Autodesk Inventor part; units mm, degrees
ref_plane "Arbeitsebene1" through (-2.597, -2.44, -3) normal (0, 0, -1) x (0, 1, 0)
ref_plane "YZ Plane" through (0, 0, 0) normal (1, 0, 0) x (0, 1, 0)
ref_plane "XZ Plane" through (0, 0, 0) normal (0, 1, 0) x (-1, 0, 0)
sketch "Skizze1" plane through (0, 0, 0) normal (0, 0, 1) x (1, 0, 0)
  circle A0 centre (11.2246, 18.4558) radius 0.3325 construction
  circle A1 centre (11.2246, 18.4558) radius 1.1
  circle A2 centre (11.2246, 18.4558) radius 2.5
  point P0 (0, 0)
  dimension "d0" = 2.2
  dimension "d1" = 5
ref_plane "Arbeitsebene1" through (-2.597, -2.44, -3) normal (0, 0, -1) x (0, 1, 0)
extrude "Extrusion1" add sketch "Skizze1" against normal up to surface (3 mm away)
sketch "Skizze2" plane through (11.2246, 18.4558, 0) normal (0, 0, 1) x (1, 0, 0)
  line L0 (0, 0) -> (-2.8913, -4.716) construction
  line L1 (-2.8913, -4.716) -> (3.5184, 5.7389) construction
  line L2 (0, 0) -> (3.8461, -2.358) construction
  line L3 (-6.9448, -1.6658) -> (-1.6658, 6.9448)
  line L4 (-1.6658, 6.9448) -> (6.9448, 1.6658)
  line L5 (6.9448, 1.6658) -> (1.6658, -6.9448)
  line L6 (1.6658, -6.9448) -> (-6.9448, -1.6658)
  line L7 (-6.9448, -1.6658) -> (6.9448, 1.6658) construction
  line L8 (-1.6658, 6.9448) -> (1.6658, -6.9448) construction
  point P0 (-11.2246, -18.4558)
  dimension "d4" = 10.1
  dimension "d5" = 10.1
extrude "Extrusion2" add sketch "Skizze2" against normal blind 2
sketch "Skizze3" plane through (0, 0, 0) normal (0, 0, 1) x (1, 0, 0)
  line L0 (4.2798, 16.79) -> (9.5588, 25.4006)
  line L1 (12.8904, 11.511) -> (4.2798, 16.79)
  line L2 (18.1694, 20.1216) -> (12.8904, 11.511)
  line L3 (9.5588, 25.4006) -> (18.1694, 20.1216)
  line L4 (4.8948, 11.5894) -> (14.4118, 5.7548)
  line L5 (14.4118, 5.7548) -> (18.7104, 12.7664)
  line L6 (18.7104, 12.7664) -> (15.0398, 15.0168)
  line L7 (-1.5402, 15.5346) -> (18.7104, 12.7664) construction
  line L8 (14.4118, 5.7548) -> (2.7585, 22.5462) construction
  line L9 (4.8948, 11.5894) -> (7.0442, 15.0952)
  line L10 (12.8904, 11.511) -> (4.2798, 16.79)
  line L11 (7.0442, 15.0952) -> (12.8904, 11.511)
  line L12 (12.8904, 11.511) -> (15.0398, 15.0168)
  line L13 (18.1694, 20.1216) -> (12.8904, 11.511)
  point P0 (0, 0)
  point P1 (8.5851, 14.1505)
extrude "Extrusion3" add sketch "Skizze3" against normal blind 6 contours L1 L2 L6 L5 L4 L9
sketch "Skizze4" plane through (4.8948, 11.5894, -6) normal (-0.5227, -0.8525, 0) x (0.8525, -0.5227, 0)
  line L0 (-1.036, 2.1441) -> (1.7865, 3.0085)
  line L1 (0, 6) -> (11.1631, 6)
  line L2 (0, 6) -> (0, 0)
  line L3 (11.1631, 0) -> (0, 0)
  line L4 (11.1631, 6) -> (11.1631, 0)
  line L5 (0.7075, 3) -> (2.9075, 3)
  line L6 (1.3376, -2.7865) -> (1.3376, -9.7615)
  ellipse E0 centre (1.3376, -6.274) end of major axis (1.3376, 3) minor radius 7.5665
  point P0 (1.8845, 6)
extrude "Extrusion4" cut sketch "Skizze4" against normal up to surface (8.2244 mm away) contours L2 E0 L0 | L2 L3 E0 | L0 E0 L3 L2
sketch "Skizze5" plane through (0, 0, 0) normal (0, 0, 1) x (1, 0, 0)
  line L0 (4.2798, 16.79) -> (9.5588, 25.4006)
  line L1 (7.0442, 15.0952) -> (4.2798, 16.79)
  line L2 (7.0442, 15.0952) -> (4.8948, 11.5894)
  line L3 (4.8948, 11.5894) -> (14.4118, 5.7548)
  line L4 (14.4118, 5.7548) -> (18.7104, 12.7664)
  line L5 (18.7104, 12.7664) -> (15.0398, 15.0168)
  line L6 (18.1694, 20.1216) -> (15.0398, 15.0168)
  line L7 (9.5588, 25.4006) -> (18.1694, 20.1216)
  line L8 (7.0442, 15.0952) -> (4.8948, 11.5894)
  line L9 (7.0442, 15.0952) -> (8.6934, 9.2606)
  line L10 (10.7856, 7.9779) -> (4.8948, 11.5894)
  point P0 (0, 0)
extrude "Extrusion5" cut sketch "Skizze5" against normal blind 6 contours L9 L3 L2
chamfer "Fase1" distance 1 angle 45 1 edges at (12.9349, 11.4837, -6)
sketch "Skizze6" plane through (14.4118, 5.7548, -6) normal (-0.5227, -0.8525, 0) x (0.8525, -0.5227, 0)
  ellipse E0 centre (-9.8255, -6.274) end of major axis (-9.8255, -15.548) minor radius 7.5665 (-4.8984, 0.7642) -> (-6.7074, 2.1759) ccw
  ellipse E1 centre (-9.8255, -6.274) end of major axis (-9.8255, -15.548) minor radius 7.5665 (-6.7074, 2.1759) -> (-11.1631, 2.8539) ccw
  point P0 (-9.2786, 6)
  point P1 (-3.2534, 0)
sketch "Skizze7" plane through (11.2246, 18.4558, -3) normal (0, 0, -1) x (-1, 0, 0)
  circle A0 centre (0, 0) radius 1.1
  point P0 (11.2246, -18.4558)
extrude "Extrusion6" cut sketch "Skizze7" against normal blind 10
properties part number "thumb_phalanx_plate" material "Nylon 6/6"
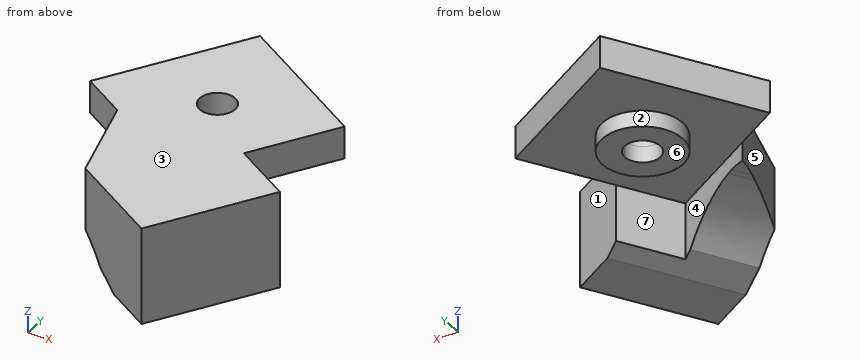
CAD build for the part. Positions are in the model's coordinates, mm. Face numbers are marked on the shaded views. A direction names the side the tool comes from. Round coordinates to 2 decimals unless told otherwise and drop trailing zeros. Write each loop counter-clockwise with the first axis right and the second up, starting at its lowest first coordinate (ties: lowest second). Pieces come first, ordered by that corner, then holes.
(1) Slice it at B-B, the plane y = 18.25. Write the cut outline in (x, z).
(2) Slice it at D-D, the plane y = 22.25. Write the cut outline in (x, z), and give its area (3 significant figures).
(3) Drop flat-ended pins along their axis: P1, Ø2, axis at y = 23, z = -1, coming from the +X side; P2, Ø2, axis at y = 18.5, z = -0.5, coming from the -X side; P3, Ø1, axis at x = 16.5, z = -4.5, coming from the +Y side. Give the stop position or say it passes through.
(4) Slice it at C-C, the plane z = -0.75. Write the cut outline in (x, y), and give its area (3 significant figures).
(5) Slice it at A-A, the plane z = -2.5. Write the cut outline in (x, y).
(6) Probe line 1 along X through (y, z) = (14.5, -2.5); line 2 along Z through (x, y) = (16, 18.75); line 3 along Y through (x, z) = (13.5, -2.75). List the from-to ranges inside material, lowest first.
(7) 3-axis set-ups, long thin cutter, end or side, ignore diameter. For the marked faces 1, 2 and 3: which of +Z, -Z, +X, -X, +Y, -Y reach the whole face in a straight line?
(8) Mould opens along X. For the marked faces 4, 5, 6 and 7 say: pulls with the +X half, pulls with the -X half, needs draft (parallel to the pull), parting line crosses it, or undercut.
From the geometry:
1. outline: (5.17, -2) - (8.73, -2) - (8.73, -3) - (10.14, -3) - (10.14, 0) - (5.17, 0) - close; (12.31, -3) - (13.72, -3) - (13.72, -2) - (17.02, -2) - (17.02, 0) - (12.31, 0) - close
2. outline: (7.63, -2) - (14.7, -2) - (14.7, 0) - (7.63, 0) - close
2. area: 14.1 mm2
3. P1: stops at x = 15.11
3. P2: stops at x = 4.72
3. P3: stops at y = 14.43
4. outline: (4.28, 16.79) - (7.04, 15.1) - (8.69, 9.26) - (14.41, 5.75) - (18.71, 12.77) - (15.04, 15.02) - (18.17, 20.12) - (9.56, 25.4) - close; hole circle Ø2.2 at (11.22, 18.46)
4. area: 153 mm2
5. outline: (7.04, 15.1) - (8.69, 9.26) - (14.41, 5.75) - (18.71, 12.77) - (15.04, 15.02) - (12.89, 11.51) - close; circle Ø5 at (11.22, 18.46); hole circle Ø2.2 at (11.22, 18.46)
6. line 1: x = 7.21 to 8.02, 14.72 to 15.88
6. line 2: z = -2 to 0
6. line 3: y = 6.31 to 12.51, 17.42 to 19.49
7. face 1: +Z, -Z, +X
7. face 2: -Z
7. face 3: +Z, +X, -X, +Y, -Y
8. face 4: undercut
8. face 5: pulls with the -X half
8. face 6: needs draft
8. face 7: undercut
